from build123d import *

# Parameters (mm, degrees)
SKETCH1_W             = 43.18
SKETCH1_H             = 38.1
BOSS_EXTRUDE1_DEPTH   = 3.175
SKETCH2_R             = 14.5
CUT_EXTRUDE1_DEPTH    = 4.175
CUT_EXTRUDE2_DEPTH    = 4.175
CIRPATTERN1_COUNT     = 3
BOSS_EXTRUDE2_DEPTH   = 3.175
CIRPATTERN2_COUNT     = 3
SKETCH6_R             = 7.62
CUT_EXTRUDE4_DEPTH    = 4.175
F_4_40_TAPPED_HOLE1_D = 2.2606


with BuildPart() as part:
    # Sketch1 → Boss-Extrude1 (new body)
    with BuildSketch(Plane.XY):
        Rectangle(SKETCH1_W, SKETCH1_H)
    extrude(amount=BOSS_EXTRUDE1_DEPTH)

    # Sketch2 → Cut-Extrude1 (cut, through all)
    with BuildSketch(Plane.XY.offset(3.175)):
        Circle(SKETCH2_R)
    extrude(amount=-CUT_EXTRUDE1_DEPTH, mode=Mode.SUBTRACT)

    # Sketch3 → Cut-Extrude2 (cut, through all)
    with BuildSketch(Plane.XY.offset(3.175)):
        with BuildLine():
            Line((-3.5, 16.63580476), (-3.5, 14.071247279))
            ThreePointArc((-3.5, 14.071247279), (0, 14.5), (3.5, 14.071247279))
            Line((3.5, 14.071247279), (3.5, 16.63580476))
            ThreePointArc((3.5, 16.63580476), (0, 17), (-3.5, 16.63580476))
        make_face()
    cut_extrude2 = extrude(amount=-CUT_EXTRUDE2_DEPTH, mode=Mode.SUBTRACT)

    # CirPattern1: Cut-Extrude2 ×3 about axis
    cirpattern1_axis = Axis((0, 0, 0), (0, 0, 1))
    for i in range(1, CIRPATTERN1_COUNT):
        add(cut_extrude2.rotate(cirpattern1_axis, i * 360 / CIRPATTERN1_COUNT), mode=Mode.SUBTRACT)

    # Sketch4 → Boss-Extrude2 (add)
    with BuildSketch(Plane.XY.offset(3.175)):
        with BuildLine():
            Line((-2.75, -13.216939888), (-2.75, -14.236836025))
            ThreePointArc((-2.75, -14.236836025), (0, -14.5), (2.75, -14.236836025))
            Line((2.75, -14.236836025), (2.75, -13.216939888))
            ThreePointArc((2.75, -13.216939888), (0, -13.5), (-2.75, -13.216939888))
        make_face()
    boss_extrude2 = extrude(amount=-BOSS_EXTRUDE2_DEPTH)

    # CirPattern2: Boss-Extrude2 ×3 about axis
    cirpattern2_axis = Axis((0, 0, 0), (0, 0, 1))
    for i in range(1, CIRPATTERN2_COUNT):
        add(boss_extrude2.rotate(cirpattern2_axis, i * 360 / CIRPATTERN2_COUNT))

    # Sketch6 → Cut-Extrude4 (cut, through all)
    with BuildSketch(Plane.XY.offset(3.175)):
        with Locations((-25.4, 0)):
            Circle(SKETCH6_R)
    extrude(amount=-CUT_EXTRUDE4_DEPTH, mode=Mode.SUBTRACT)

    # #4-40 Tapped Hole1 (through all)
    with Locations(Plane(origin=(0, 0, 0), x_dir=(-1, 0, 0), z_dir=(0, 0, -1))):
        with Locations((-17.78, 15.24), (-17.78, -8.89), (17.78, -8.89), (17.78, 15.24)):
            Hole(F_4_40_TAPPED_HOLE1_D / 2)


solid = part.part
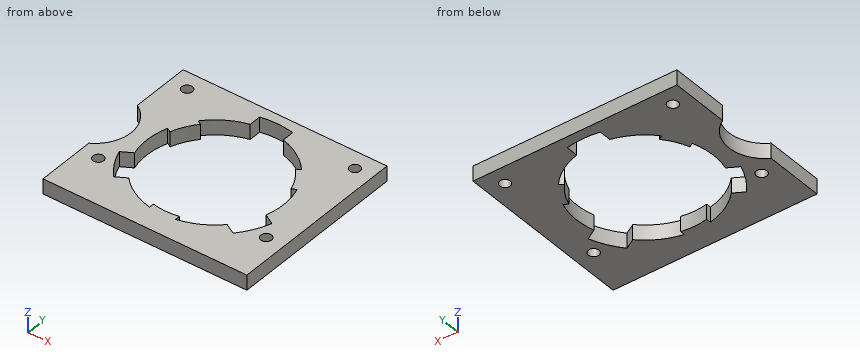
The listing builds one solid part. Answer for the finished solid, in the listing's coordinates (mm). Coordinates: 2 decimals unless noted, no trailing zeros. Write each loop counter-clockwise with the first axis right and the second up, starting at its lowest first coordinate (ties: lowest second). Pieces come first, ordered by that corner, then holes. Notation, with made-up numbers: (-3.5, -9.5) - (49.5, -9.5) arc R34 cw to (49.5, 22.5) - close; hole circle Ø6 at (6, 68.25). An arc over 180 degrees is marked (long way). Return JSON: item names as keys, results as strings.
1. The part is cut by section B-B on x = 17.78. Determine the outline of the cut face in (y, z) (3 decimals).
Final values:
{"outline": "(-19.05, 0) - (-10.02, 0) - (-10.02, 3.175) - (-19.05, 3.175) - close; (-7.76, 0) - (14.11, 0) - (14.11, 3.175) - (-7.76, 3.175) - close; (16.37, 0) - (19.05, 0) - (19.05, 3.175) - (16.37, 3.175) - close"}
2. Consider line 1 along Y through (x, z) = (17.78, 1.75); line 2 along Y through (x, z) = (18, 2.6); line 3 along Y through (x, z) = (4, 2.85). Determine where each line is inside the solid, lowest interval first.
Final values:
{"line 1": "-19.05 to -10.02, -7.76 to 14.11, 16.37 to 19.05", "line 2": "-19.05 to -10, -7.78 to 14.13, 16.35 to 19.05", "line 3": "-19.05 to -13.94, 13.94 to 19.05"}
3. The part is cut by section C-C on y = 13.5. Determine the outline of the cut face in (x, z) (1 decimal), then the cut area to 3 significant figures.
Final values:
{"outline": "(-21.6, 0) - (-5.3, 0) - (-5.3, 3.2) - (-21.6, 3.2) - close; (5.3, 0) - (21.6, 0) - (21.6, 3.2) - (5.3, 3.2) - close", "area": "103 mm^2"}
4. The part is cut by section A-A on z = 1.5. Count the separate pieces of the cut face and the enclosed holes in it, then the cut area to 3 significant figures.
Final values:
{"separate pieces": "1", "enclosed holes": "5", "area": "897 mm^2"}
5. The part is cut by section D-D on x = 12. Determine the outline of the cut face in (y, z) (3 decimals), then the cut area to 3 significant figures.
Final values:
{"outline": "(-19.05, 0) - (-10.97, 0) - (-10.97, 3.175) - (-19.05, 3.175) - close; (6.185, 0) - (19.05, 0) - (19.05, 3.175) - (6.185, 3.175) - close", "area": "66.5 mm^2"}
